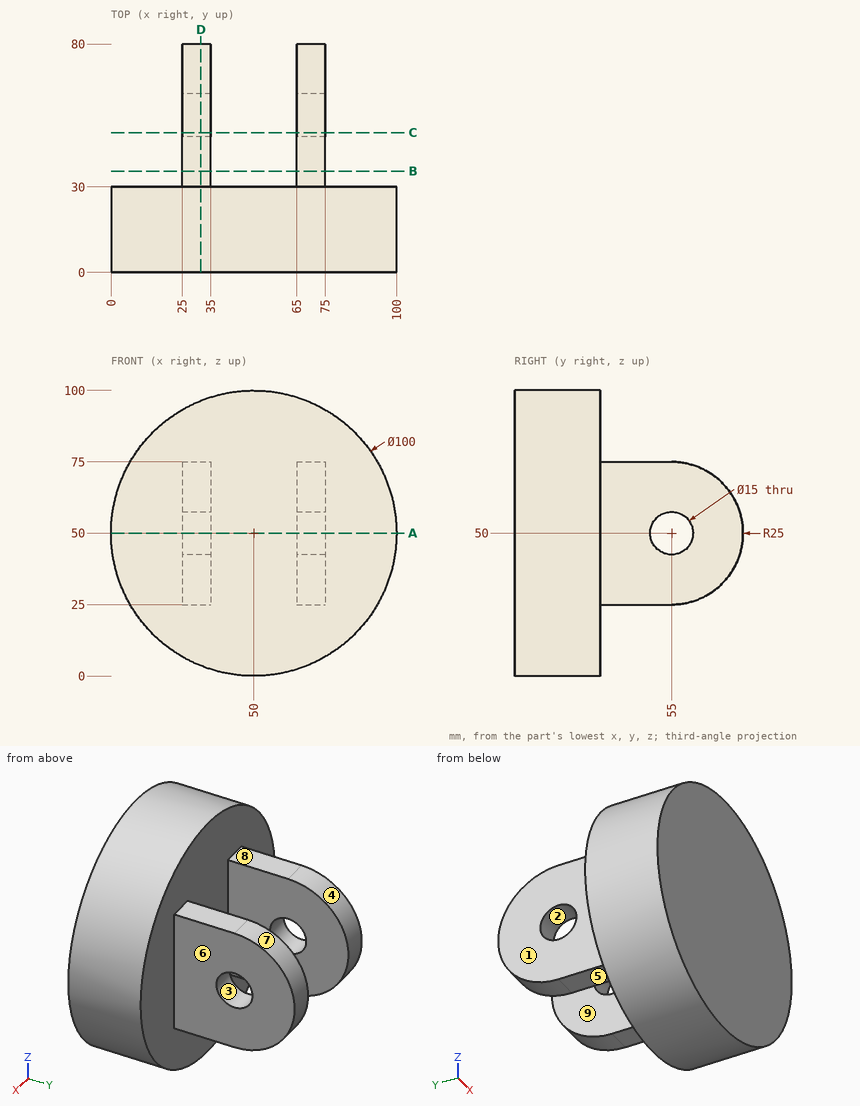
Print and shaded views of the part. All mm, measured from the part's lowest x, y and z. A direction names the side the tool comes from. Round coordinates to 2 decimals unless told otherwise and drop trailing zeros. Write each loop counter-clockwise with the first axis right and the second up, starting at its lowest first coordinate (ties: lowest second). Pieces come first, ordered by that corner, then holes. Notation, with made-up numbers: M 48,31.5 L 107,31.5 A20 cw 107,62.5 Z; hole C -11,-36 d1. An arc over 180 degrees is marked long. Use a Markdown table: item, result. Add a question column.
1. Slice it at C-C on y = 49. Give the cut face in (x, z).
2. Slice it at A-A on z = 50. Give the cut face in (x, y).
3. Slice it at D-D on x = 31.5. Give the cut face in (y, z).
4. 3-axis set-ups, long thin cutter, end or side, ignore diameter. For the marked faces 5, 6, 7, 8 and 9: which of +Z, -Z, +X, -X, +Y, -Y reach the whole face in a straight line?
5. Slice it at B-B on y = 35.5. Give the cut face in (x, z), then the cut area to 3 significant figures.
6. Drill centre lines: probe 1 along X at (y, z) = (35.5, 36.5); probe 2 along Y at (x, z) = (70, 50); probe 3 along Y at (x, z) = (70, 89). Where is each one in solid material? Low to high.
7. Flat gauge pins, fed straight in: P1, Ø1, axis at x = 77.5, z = 54.5, coming from the -Y side; P2, Ø3, axis at y = 39, z = 71.5, coming from the -X side; P3, Ø5, axis at y = 46, z = 67.5, coming from the +X side; P4, Ø3, axis at x = 28.5, y = 41.5, coming from the +Z side. Where does each tip first touch, or does it go through?
8. Pull direction Z, two halves, no side cores. Call the marked faces 1, 2, 3 and 4: released by +Z, released by -Z, zero draft, split by the parting line, or undercut.
Reply:
| question | item | result |
|---|---|---|
| 1 | outline | M 25,25 L 35,25 L 35,45.5 L 25,45.5 Z; M 25,54.5 L 35,54.5 L 35,75 L 25,75 Z; M 65,25 L 75,25 L 75,45.5 L 65,45.5 Z; M 65,54.5 L 75,54.5 L 75,75 L 65,75 Z |
| 2 | outline | M 0,0 L 100,0 L 100,30 L 75,30 L 75,47.5 L 65,47.5 L 65,30 L 35,30 L 35,47.5 L 25,47.5 L 25,30 L 0,30 Z; M 25,62.5 L 35,62.5 L 35,80 L 25,80 Z; M 65,62.5 L 75,62.5 L 75,80 L 65,80 Z |
| 3 | outline | M 0,3.55 L 30,3.55 L 30,25 L 55,25 A25 ccw 55,75 L 30,75 L 30,96.45 L 0,96.45 Z; hole C 55,50 d15 |
| 4 | face 5 | -Z, +X, -X, +Y |
| 4 | face 6 | +Z, -Z, +X, +Y |
| 4 | face 7 | +X, -X, +Y |
| 4 | face 8 | +Z, +X, -X, +Y |
| 4 | face 9 | +Z, -Z, +Y |
| 5 | outline | M 25,25 L 35,25 L 35,75 L 25,75 Z; M 65,25 L 75,25 L 75,75 L 65,75 Z |
| 5 | area | 1,000 mm^2 |
| 6 | probe 1 | x = 25 to 35, 65 to 75 |
| 6 | probe 2 | y = 0 to 47.5, 62.5 to 80 |
| 6 | probe 3 | y = 0 to 30 |
| 7 | P1 | stops at y = 0 |
| 7 | P2 | stops at x = 25 |
| 7 | P3 | stops at x = 75 |
| 7 | P4 | stops at z = 75 |
| 8 | face 1 | zero draft |
| 8 | face 2 | undercut |
| 8 | face 3 | undercut |
| 8 | face 4 | split by the parting line |
